For this review, take the finished solid that the model builds, in its own axes (mm). Round coordinates to 2 decimals unless told otherwise and drop trailing zeros. Write each loop counter-clockwise with the first axis right and the second up, starting at its lowest first coordinate (ties: lowest second). Pieces come first, ordered by that corner, then holes. Notation, with made-up numbers: M -39,52 L -31,52 A34 cw -31,88 Z; hole C 57,-30 d1. An arc over 180 degrees is marked long. Answer in a Markdown table with one row per item.
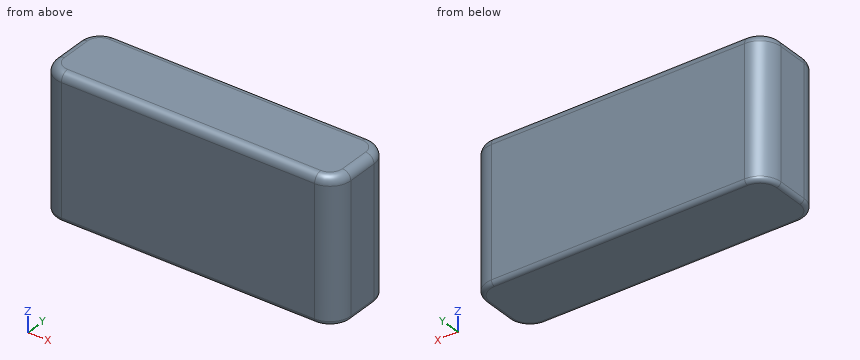
```python
from build123d import *

# Parameters (mm, degrees)
SKETCH1_W           = 71
SKETCH1_H           = 34
BOSS_EXTRUDE1_DEPTH = 17.5
FILLET1_R           = 5
FILLET2_R           = 2
FILLET3_R           = 1


with BuildPart() as part:
    # Sketch1 → Boss-Extrude1 (new body)
    with BuildSketch(Plane(origin=(0, 0, 0), x_dir=(1, 0, 0), z_dir=(0, 1, 0))):
        Rectangle(SKETCH1_W, SKETCH1_H)
    extrude(amount=BOSS_EXTRUDE1_DEPTH)

    # Fillet1
    fillet1_edges = [part.edges().sort_by_distance(p)[0] for p in [
        (35.5, 17.5, 0),
        (-35.5, 17.5, 0),
        (35.5, 0, 0),
        (-35.5, 0, 0),
    ]]
    fillet(fillet1_edges, radius=FILLET1_R)

    # Fillet2
    fillet2_edges = [part.edges().sort_by_distance(p)[0] for p in [
        (-35.5, 8.75, 17),
        (0, 0, 17),
        (35.5, 8.75, 17),
        (0, 17.5, 17),
        (-34.035533906, 16.035533906, 17),
        (34.035533906, 16.035533906, 17),
        (34.035533906, 1.464466094, 17),
        (-34.035533906, 1.464466094, 17),
    ]]
    fillet(fillet2_edges, radius=FILLET2_R)

    # Fillet3
    fillet3_edges = [part.edges().sort_by_distance(p)[0] for p in [
        (-35.5, 8.75, -17),
        (0, 0, -17),
        (0, 17.5, -17),
        (35.5, 8.75, -17),
        (-34.035533906, 16.035533906, -17),
        (34.035533906, 16.035533906, -17),
        (34.035533906, 1.464466094, -17),
        (-34.035533906, 1.464466094, -17),
    ]]
    fillet(fillet3_edges, radius=FILLET3_R)


solid = part.part
```
Q1. Take a section at A-A (z = 7.5). State the section outline as (x, y) points.
Found:
| item | result |
|---|---|
| outline | M -35.5,5 A5 ccw -30.5,0 L 30.5,0 A5 ccw 35.5,5 L 35.5,12.5 A5 ccw 30.5,17.5 L -30.5,17.5 A5 ccw -35.5,12.5 Z |
Q2. For probe 1 along Z at (x, y) = (12, 15.75); probe 2 along X at (y, z) = (1.25, -12.5); probe 3 along X at (y, z) = (15.75, -3.5), list the stretches that pass through material, from the lowest coordinate up.
Found:
| item | result |
|---|---|
| probe 1 | -17 to 16.98 |
| probe 2 | -33.81 to 33.81 |
| probe 3 | -34.3 to 34.3 |
Q3. Insertion check: P1, Ø5, axis at y = 3, z = 12.5, coming from the -X side; P2, Ø1.5, axis at y = 14, z = 11.5, coming from the -X side. Each pin has a flat end and moves straight along its axis. Give the tip position at first contact, or say it passes through.
Found:
| item | result |
|---|---|
| P1 | x = -35.5 |
| P2 | x = -35.44 |
